The model under review builds one solid part; all positions refer to its coordinate system, in mm. A direction names the side the tool comes from. Round coordinates to 2 decimals unless told otherwise and drop trailing zeros. Write each loop counter-clockwise with the first axis right and the second up, starting at its lowest first coordinate (ties: lowest second). Pieces come first, ordered by that corner, then holes. Notation, with made-up numbers: (-19.75, -19.5) - (11.25, -19.5) arc R28 cw to (11.25, 16.5) - close; hole circle Ø10 at (-11, 25.5). An arc over 180 degrees is marked (long way). Return JSON: item names as keys, results as strings.
from build123d import *

# Parameters (mm, degrees)
F1_DEPTH     = 3
F2_T1_DEPTH  = 69.0608621697
F2_T3_DEPTH  = 65.2081986538
F2_T5_DEPTH  = 71.5756555765
F2_T7_DEPTH  = 30.9128784748
F2_T9_DEPTH  = 38.9128784748
F2_T11_DEPTH = 35.9128784748
F2_T13_DEPTH = 40.9128784748
F2_T15_DEPTH = 40.9128784748
F2_T17_DEPTH = 35.9128784748


# Not quite as in the source:
# - a fillet or chamfer that OpenCascade refuses, or shapes differently, is made with other operations: its cross-section is extruded or revolved along the edge and cut away or added


with BuildPart() as f1:
    # F0 (on Front) → F1 (new body)
    with BuildSketch(Plane.XZ):
        with BuildLine():
            Line((-39.3023127707, 0), (-39.3023127707, -40.6627771018))
            Line((-39.3023127707, -40.6627771018), (-9.0223597329, -40.6627771018))
            ThreePointArc((-9.0223597329, -40.6627771018), (-6.6956927949, -15.256923351), (15, -28.6795794964))
            ThreePointArc((15, -28.6795794964), (13.4226561454, -35.3752722912), (9.0223597329, -40.6627771018))
            Line((9.0223597329, -40.6627771018), (34.6976872293, -40.6627771018))
            Line((34.6976872293, -40.6627771018), (34.6976872293, 0))
            Line((34.6976872293, 0), (34.6976872293, 8))
            Line((34.6976872293, 8), (29.6976872293, 8))
            Line((29.6976872293, 8), (29.6976872293, 12))
            Line((29.6976872293, 12), (34.6976872293, 12))
            Line((34.6976872293, 12), (34.6976872293, 20))
            Line((34.6976872293, 20), (29.6976872293, 20))
            Line((29.6976872293, 20), (29.6976872293, 24))
            Line((29.6976872293, 24), (34.6976872293, 24))
            Line((34.6976872293, 24), (34.6976872293, 40))
            Line((34.6976872293, 40), (21.6976872293, 40))
            Line((21.6976872293, 40), (21.6976872293, 35))
            Line((21.6976872293, 35), (17.6976872293, 35))
            Line((17.6976872293, 35), (17.6976872293, 40))
            Line((17.6976872293, 40), (-0.3023127707, 40))
            Line((-0.3023127707, 40), (-0.3023127707, 35))
            Line((-0.3023127707, 35), (-4.3023127707, 35))
            Line((-4.3023127707, 35), (-4.3023127707, 40))
            Line((-4.3023127707, 40), (-22.3023127707, 40))
            Line((-22.3023127707, 40), (-22.3023127707, 35))
            Line((-22.3023127707, 35), (-26.3023127707, 35))
            Line((-26.3023127707, 35), (-26.3023127707, 40))
            Line((-26.3023127707, 40), (-39.3023127707, 40))
            Line((-39.3023127707, 40), (-39.3023127707, 24))
            Line((-39.3023127707, 24), (-34.3023127707, 24))
            Line((-34.3023127707, 24), (-34.3023127707, 20))
            Line((-34.3023127707, 20), (-39.3023127707, 20))
            Line((-39.3023127707, 20), (-39.3023127707, 12))
            Line((-39.3023127707, 12), (-34.3023127707, 12))
            Line((-34.3023127707, 12), (-34.3023127707, 8))
            Line((-34.3023127707, 8), (-39.3023127707, 8))
            Line((-39.3023127707, 8), (-39.3023127707, 0))
        make_face()
        with BuildLine():
            ThreePointArc((-31.7284863554, 20), (-20.5985922366, 31.1298941188), (-9.4686981178, 20))
            Line((-9.4686981178, 20), (-20.5985922366, 8))
            Line((-20.5985922366, 8), (-31.7284863554, 20))
        make_face(mode=Mode.SUBTRACT)
        with BuildLine():
            ThreePointArc((4.2398196727, 20), (14.8943690583, 30.6545493856), (25.5489184439, 20))
            Line((25.5489184439, 20), (14.8943690583, 8))
            Line((14.8943690583, 8), (4.2398196727, 20))
        make_face(mode=Mode.SUBTRACT)
        with BuildLine():
            Line((-9.0223597329, -40.6627771018), (-39.3023127707, -40.6627771018))
            Line((-39.3023127707, -40.6627771018), (0, -64.8488187371))
            Line((0, -64.8488187371), (34.6976872293, -40.6627771018))
            Line((34.6976872293, -40.6627771018), (9.0223597329, -40.6627771018))
            ThreePointArc((9.0223597329, -40.6627771018), (0, -43.6795794964), (-9.0223597329, -40.6627771018))
        make_face()
    extrude(amount=F1_DEPTH)

    # F2: fillet of radius 5 on 12 edges, made by hand

    # F2_s2 → F2_t1 (cut)
    with BuildSketch(Plane(origin=(-20.1138870842, 0, 12.3777782062), x_dir=(0, 1, 0), z_dir=(0.8516582876, 0, -0.5240974729))):
        with BuildLine():
            ThreePointArc((0, -55.2290339197), (-2.1833001327, -53.3850710123), (-3, -50.6464582247))
            Line((-3, -50.6464582247), (-3, -55.2290339197))
            Line((-3, -55.2290339197), (0, -55.2290339197))
        make_face()
    extrude(amount=F2_T1_DEPTH, mode=Mode.SUBTRACT)

    # F2_s4 → F2_t3 (cut)
    with BuildSketch(Plane(origin=(-39.8201349052, 0, -27.7566465561), x_dir=(0, 1, 0), z_dir=(0.8203670544, 0, 0.5718372986))):
        with BuildLine():
            ThreePointArc((0, -53.1998344073), (-2.1833001327, -51.3558714999), (-3, -48.6172587124))
            Line((-3, -48.6172587124), (-3, -53.1998344073))
            Line((-3, -53.1998344073), (0, -53.1998344073))
        make_face()
    extrude(amount=F2_T3_DEPTH, mode=Mode.SUBTRACT)

    # F2_s6 → F2_t5 (cut)
    with BuildSketch(Plane.XY.offset(-52.1192163392)):
        with BuildLine():
            ThreePointArc((-39.3023127707, 0), (-37.4583498632, -2.1833001327), (-34.7197370757, -3))
            Line((-34.7197370757, -3), (-39.3023127707, -3))
            Line((-39.3023127707, -3), (-39.3023127707, 0))
        make_face()
        with BuildLine():
            ThreePointArc((34.6976872293, 0), (32.8537243219, -2.1833001327), (30.1151115344, -3))
            Line((30.1151115344, -3), (34.6976872293, -3))
            Line((34.6976872293, -3), (34.6976872293, 0))
        make_face()
    extrude(amount=F2_T5_DEPTH, mode=Mode.SUBTRACT)

    # F2_s8 → F2_t7 (cut)
    with BuildSketch(Plane.XY.offset(0.5435607626)):
        with BuildLine():
            ThreePointArc((-39.3023127707, 0), (-37.4583498632, -2.1833001327), (-34.7197370757, -3))
            Line((-34.7197370757, -3), (-39.3023127707, -3))
            Line((-39.3023127707, -3), (-39.3023127707, 0))
        make_face()
        with BuildLine():
            ThreePointArc((34.6976872293, 0), (32.8537243219, -2.1833001327), (30.1151115344, -3))
            Line((30.1151115344, -3), (34.6976872293, -3))
            Line((34.6976872293, -3), (34.6976872293, 0))
        make_face()
    extrude(amount=F2_T7_DEPTH, mode=Mode.SUBTRACT)

    # F2_s10 → F2_t9 (cut)
    with BuildSketch(Plane.XY.offset(12.5435607626)):
        with BuildLine():
            ThreePointArc((-39.3023127707, 0), (-37.4583498632, -2.1833001327), (-34.7197370757, -3))
            Line((-34.7197370757, -3), (-39.3023127707, -3))
            Line((-39.3023127707, -3), (-39.3023127707, 0))
        make_face()
        with BuildLine():
            ThreePointArc((34.6976872293, 0), (32.8537243219, -2.1833001327), (30.1151115344, -3))
            Line((30.1151115344, -3), (34.6976872293, -3))
            Line((34.6976872293, -3), (34.6976872293, 0))
        make_face()
    extrude(amount=F2_T9_DEPTH, mode=Mode.SUBTRACT)

    # F2_s12 → F2_t11 (cut)
    with BuildSketch(Plane.YZ.offset(-50.7587520081)):
        with BuildLine():
            ThreePointArc((0, 40), (-2.1833001327, 38.1560370926), (-3, 35.417424305))
            Line((-3, 35.417424305), (-3, 40))
            Line((-3, 40), (0, 40))
        make_face()
    extrude(amount=F2_T11_DEPTH, mode=Mode.SUBTRACT)

    # F2_s14 → F2_t13 (cut)
    with BuildSketch(Plane.YZ.offset(-33.7587520081)):
        with BuildLine():
            ThreePointArc((0, 40), (-2.1833001327, 38.1560370926), (-3, 35.417424305))
            Line((-3, 35.417424305), (-3, 40))
            Line((-3, 40), (0, 40))
        make_face()
    extrude(amount=F2_T13_DEPTH, mode=Mode.SUBTRACT)

    # F2_s16 → F2_t15 (cut)
    with BuildSketch(Plane.YZ.offset(-11.7587520081)):
        with BuildLine():
            ThreePointArc((0, 40), (-2.1833001327, 38.1560370926), (-3, 35.417424305))
            Line((-3, 35.417424305), (-3, 40))
            Line((-3, 40), (0, 40))
        make_face()
    extrude(amount=F2_T15_DEPTH, mode=Mode.SUBTRACT)

    # F2_s18 → F2_t17 (cut)
    with BuildSketch(Plane.YZ.offset(10.2412479919)):
        with BuildLine():
            ThreePointArc((0, 40), (-2.1833001327, 38.1560370926), (-3, 35.417424305))
            Line((-3, 35.417424305), (-3, 40))
            Line((-3, 40), (0, 40))
        make_face()
    extrude(amount=F2_T17_DEPTH, mode=Mode.SUBTRACT)


solid = f1.part
(1) Wall thickness on line 1 (Z direction, x = 5.5, y = -1.3); line 2 (X direction, y = -1.7, z = 25.5); line 3 (X direction, y = -0.3, z = 24.5): over which ranges is each line inside the solid? List them lowest first.
Filled in:
{"line 1": "z = -60.01 to -42.63, -14.72 to 18.58, 25.03 to 39.17", "line 2": "x = -38.08 to -30.27, -10.92 to 5.77, 24.02 to 33.48", "line 3": "x = -39.16 to -30.78, -10.42 to 5.24, 24.55 to 34.55"}
(2) Add section A-A (z = -33.5). Write out the cut boundary in (x, y), plus the area to 3 significant figures.
Filled in:
{"outline": "(-39.3, 0) arc R5 ccw to (-34.72, -3) - (-14.2, -3) - (-14.2, 0) - close; (14.2, -3) - (30.12, -3) arc R5 ccw to (34.7, 0) - (14.2, 0) - close", "area": "129 mm2"}
(3) For faces 5 (the cylindrical face through (-13.43, -2.16, 38.19)), 6 (the flat face through (-36, -1, 20)), 7 (the flat face through (32, -1, 12)), 8 (the flat face through (-22.302, -1, 37)), 9 (the cylindrical face through (14.66, -1.48, 30.65)), list the 3-axis set-ups (+Z, -Z, +X, -X, +Y, -Y) from which the entire face can be reached by the end or side of a thin tool; tool diameter is ignored.
Filled in:
{"face 5": "+Z, +X, -X, -Y", "face 6": "-X, +Y, -Y", "face 7": "+X, +Y, -Y", "face 8": "+Z, +Y, -Y", "face 9": "+Y, -Y"}
(4) Add section C-C (y = -1.95). Give the number of separate pieces and of enclosed holes in the cut face, plus the area to 3 significant figures.
Filled in:
{"separate pieces": "1", "enclosed holes": "3", "area": "4,940 mm2"}
(5) Mouldability with a two-part tool opening along Z and no side actions: class faces 1 (the flat face through (-2, -1, 35)), 2 (the flat face through (32, -1, 8)), 3 (the cylindrical face through (32.89, -2.16, 15.94)), 4 (the flat face through (32, -1, 20)) as released by +Z, released by -Z, zero draft, split by the parting line, or undercut.
Filled in:
{"face 1": "released by +Z", "face 2": "undercut", "face 3": "zero draft", "face 4": "undercut"}
(6) Clearance check with flat-ended pins moving along their axes: pin 1 Ø1.5 at (x, y) = (-2.5, -1) entering from +Z; pin 2 Ø0.9 at (y, z) = (-2, 37.5) entering from +X; pin 3 Ø0.9 at (y, z) = (-1, 22) entering from -X. State where each tip first meets the part, or that it passes through.
Filled in:
{"pin 1": "stops at z = 35", "pin 2": "stops at x = 33.64", "pin 3": "stops at x = -34.3"}
(7) Add section B-B (z = 16). Write out the cut boundary in (x, y).
Filled in:
{"outline": "(-39.3, 0) arc R5 ccw to (-34.72, -3) - (-28.02, -3) - (-28.02, 0) - close; (-13.18, -3) - (7.79, -3) - (7.79, 0) - (-13.18, 0) - close; (22, -3) - (30.12, -3) arc R5 ccw to (34.7, 0) - (22, 0) - close"}
